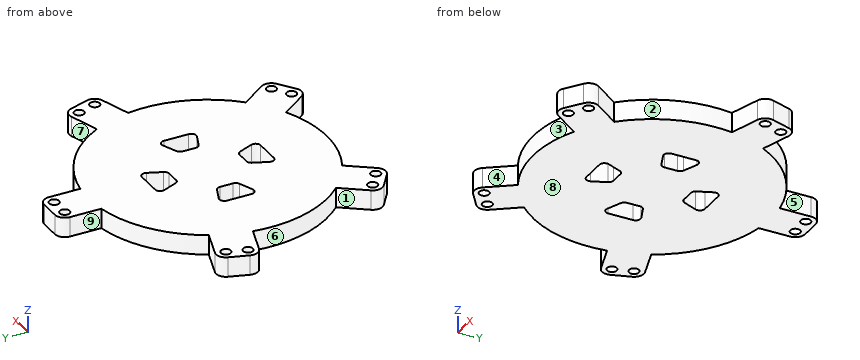
from build123d import *

# Parameters (mm, degrees)
F0_R     = 1.5875
F1_DEPTH = 6.3754
F3_DEPTH = 6.3764


with BuildPart() as f1:
    # F0 (on Top) → F1 (new body)
    with BuildSketch(Plane.XY):
        with BuildLine():
            Line((-6.35, 47.625), (-6.35, 37.567107))
            ThreePointArc((-6.35, 37.567107), (-22.394618, 30.823547), (-33.766184, 17.648083))
            Line((-33.766184, 17.648083), (-43.331809, 20.756143))
            ThreePointArc((-43.331809, 20.756143), (-45.754357, 20.565485), (-47.332542, 18.717668))
            Line((-47.332542, 18.717668), (-49.2948, 12.678459))
            ThreePointArc((-49.2948, 12.678459), (-49.104141, 10.25591), (-47.256325, 8.677725))
            Line((-47.256325, 8.677725), (-37.690699, 5.569665))
            ThreePointArc((-37.690699, 5.569665), (-36.235253, -11.773547), (-27.218649, -26.659991))
            Line((-27.218649, -26.659991), (-33.130531, -34.796998))
            ThreePointArc((-33.130531, -34.796998), (-33.697812, -37.159896), (-32.42812, -39.231845))
            Line((-32.42812, -39.231845), (-27.290862, -42.964281))
            ThreePointArc((-27.290862, -42.964281), (-24.927964, -43.531563), (-22.856015, -42.261871))
            Line((-22.856015, -42.261871), (-16.944133, -34.124864))
            ThreePointArc((-16.944133, -34.124864), (0, -38.1), (16.944133, -34.124864))
            Line((16.944133, -34.124864), (22.856015, -42.261871))
            ThreePointArc((22.856015, -42.261871), (24.927964, -43.531563), (27.290862, -42.964281))
            Line((27.290862, -42.964281), (32.42812, -39.231845))
            ThreePointArc((32.42812, -39.231845), (33.697812, -37.159896), (33.130531, -34.796998))
            Line((33.130531, -34.796998), (27.218649, -26.659991))
            ThreePointArc((27.218649, -26.659991), (36.235253, -11.773547), (37.690699, 5.569665))
            Line((37.690699, 5.569665), (47.256325, 8.677725))
            ThreePointArc((47.256325, 8.677725), (49.104141, 10.25591), (49.2948, 12.678459))
            Line((49.2948, 12.678459), (47.332542, 18.717668))
            ThreePointArc((47.332542, 18.717668), (45.754357, 20.565485), (43.331809, 20.756143))
            Line((43.331809, 20.756143), (33.766184, 17.648083))
            ThreePointArc((33.766184, 17.648083), (22.394618, 30.823547), (6.35, 37.567107))
            Line((6.35, 37.567107), (6.35, 47.625))
            ThreePointArc((6.35, 47.625), (5.420064, 49.870064), (3.175, 50.8))
            Line((3.175, 50.8), (-3.175, 50.8))
            ThreePointArc((-3.175, 50.8), (-5.420064, 49.870064), (-6.35, 47.625))
        make_face()
        with Locations((-25.424644, -40.395653)):
            Circle(F0_R, mode=Mode.SUBTRACT)
        with Locations((-30.561902, -36.663216)):
            Circle(F0_R, mode=Mode.SUBTRACT)
        with Locations((25.424644, -40.395653)):
            Circle(F0_R, mode=Mode.SUBTRACT)
        with Locations((30.561902, -36.663216)):
            Circle(F0_R, mode=Mode.SUBTRACT)
        with Locations((-46.275196, 11.69733)):
            Circle(F0_R, mode=Mode.SUBTRACT)
        with Locations((-44.312938, 17.736539)):
            Circle(F0_R, mode=Mode.SUBTRACT)
        with Locations((-3.175, 47.625)):
            Circle(F0_R, mode=Mode.SUBTRACT)
        with Locations((46.275196, 11.69733)):
            Circle(F0_R, mode=Mode.SUBTRACT)
        with Locations((44.312938, 17.736539)):
            Circle(F0_R, mode=Mode.SUBTRACT)
        with Locations((3.175, 47.625)):
            Circle(F0_R, mode=Mode.SUBTRACT)
    extrude(amount=F1_DEPTH)

    # F2 (on face) → F3 (cut, through all)
    with BuildSketch(Plane.XY.offset(6.3754)):
        with BuildLine():
            Line((3.984938, 19.05), (0, 19.05))
            Line((0, 19.05), (-3.984938, 19.05))
            ThreePointArc((-3.984938, 19.05), (-5.303035, 18.347246), (-5.454143, 16.861174))
            Line((-5.454143, 16.861174), (-3.578628, 12.278771))
            ThreePointArc((-3.578628, 12.278771), (-2.994169, 11.562), (-2.109423, 11.292597))
            Line((-2.109423, 11.292597), (0, 11.292597))
            Line((0, 11.292597), (2.109423, 11.292597))
            ThreePointArc((2.109423, 11.292597), (2.994169, 11.562), (3.578628, 12.278771))
            Line((3.578628, 12.278771), (5.454143, 16.861174))
            ThreePointArc((5.454143, 16.861174), (5.303035, 18.347246), (3.984938, 19.05))
        make_face()
        with BuildLine():
            Line((19.05, -3.984938), (19.05, 0))
            Line((19.05, 0), (19.05, 3.984938))
            ThreePointArc((19.05, 3.984938), (18.347246, 5.303035), (16.861174, 5.454143))
            Line((16.861174, 5.454143), (12.278771, 3.578628))
            ThreePointArc((12.278771, 3.578628), (11.562, 2.994169), (11.292597, 2.109423))
            Line((11.292597, 2.109423), (11.292597, 0))
            Line((11.292597, 0), (11.292597, -2.109423))
            ThreePointArc((11.292597, -2.109423), (11.562, -2.994169), (12.278771, -3.578628))
            Line((12.278771, -3.578628), (16.861174, -5.454143))
            ThreePointArc((16.861174, -5.454143), (18.347246, -5.303035), (19.05, -3.984938))
        make_face()
        with BuildLine():
            Line((-3.984938, -19.05), (0, -19.05))
            Line((0, -19.05), (3.984938, -19.05))
            ThreePointArc((3.984938, -19.05), (5.303035, -18.347246), (5.454143, -16.861174))
            Line((5.454143, -16.861174), (3.578628, -12.278771))
            ThreePointArc((3.578628, -12.278771), (2.994169, -11.562), (2.109423, -11.292597))
            Line((2.109423, -11.292597), (0, -11.292597))
            Line((0, -11.292597), (-2.109423, -11.292597))
            ThreePointArc((-2.109423, -11.292597), (-2.994169, -11.562), (-3.578628, -12.278771))
            Line((-3.578628, -12.278771), (-5.454143, -16.861174))
            ThreePointArc((-5.454143, -16.861174), (-5.303035, -18.347246), (-3.984938, -19.05))
        make_face()
        with BuildLine():
            Line((-19.05, 3.984938), (-19.05, 0))
            Line((-19.05, 0), (-19.05, -3.984938))
            ThreePointArc((-19.05, -3.984938), (-18.347246, -5.303035), (-16.861174, -5.454143))
            Line((-16.861174, -5.454143), (-12.278771, -3.578628))
            ThreePointArc((-12.278771, -3.578628), (-11.562, -2.994169), (-11.292597, -2.109423))
            Line((-11.292597, -2.109423), (-11.292597, 0))
            Line((-11.292597, 0), (-11.292597, 2.109423))
            ThreePointArc((-11.292597, 2.109423), (-11.562, 2.994169), (-12.278771, 3.578628))
            Line((-12.278771, 3.578628), (-16.861174, 5.454143))
            ThreePointArc((-16.861174, 5.454143), (-18.347246, 5.303035), (-19.05, 3.984938))
        make_face()
    extrude(amount=-F3_DEPTH, mode=Mode.SUBTRACT)


solid = f1.part
The listing builds one solid part. Answer for the finished solid, in the listing's coordinates (mm). Face numbers are marked on the shaded views. A direction names the side the tool comes from. Give positions to 0.01 mm unless a question says otherwise; leave off trailing zeros. Order: outer loops, then holes, each group sorted by start corner. A loop starts at its lowest first (then second) coordinate and runs counter-clockwise, first axis right, second up. Notation, with made-up numbers: (78, 22) -> (127, 22) arc R17 ccw to (127, 36) -> close; hole circle Ø1 at (63.25, -32.75). An arc over 180 degrees is marked (long way). Put each result on its own line as item: value.
Item 1: For the marked faces 5, 6, 7, 8 and 9, determine the directions among +Z, -Z, +X, -X, +Y, -Y from which every point of the face is accessible in a straight line to the end or side of a thin tool.
Established:
face 5: +Z, -Z, +X, +Y
face 6: +Z, -Z, -X
face 7: +Z, -Z, +Y
face 8: -Z, +X, -X, +Y, -Y
face 9: +Z, -Z, -X, +Y
Item 2: A cutting plane is placed at D-D on y = -22. Give the vertices of the cut face in (x, z).
Established:
outline: (-31.11, 0) -> (31.11, 0) -> (31.11, 6.38) -> (-31.11, 6.38) -> close
Item 3: A cutting plane is placed at C-C on z = 3.5. Count the separate pieces of the cut face and the enclosed holes in it, plus the area to 3 significant figures.
Established:
separate pieces: 1
enclosed holes: 14
area: 4,990 mm^2
Item 4: A cutting plane is placed at B-B on y = 42.5. Give the vertices of the cut face in (x, z), plus the area to 3 significant figures.
Established:
outline: (-6.35, 0) -> (6.35, 0) -> (6.35, 6.38) -> (-6.35, 6.38) -> close
area: 81.0 mm^2
Item 5: A cutting plane is placed at A-A on x = 15. Give the vertices of the cut face in (y, z), plus the area to 3 significant figures.
Established:
outline: (-35.02, 0) -> (-4.69, 0) -> (-4.69, 6.38) -> (-35.02, 6.38) -> close; (4.69, 0) -> (35.02, 0) -> (35.02, 6.38) -> (4.69, 6.38) -> close
area: 387 mm^2
Item 6: Given P1, Ø1, axis at x = 1.5, z = 2.5, coming from the -Y side; P2, Ø2, axis at y = 0, z = 2.5, coming from the -X side; P3, Ø3.5, axis at y = -1, z = 2.5, coming from the +X side, each flat-ended and moving along its own axis, determine where each tip first touches the part or whether it passes through.
Established:
P1: stops at y = -38.09
P2: stops at x = -38.1
P3: stops at x = 38.1
Item 7: For a pull along X with two mould halves and no side action, classify the marked faces 1, 2, 3 and 4 as released by +X, released by -X, zero draft, split by the parting line, or undercut.
Established:
face 1: released by -X
face 2: released by +X
face 3: undercut
face 4: undercut
Item 8: Straight lines are drawn through the part: line 1 (X direction, y = 1, z = 5.5); line 2 (Y direction, x = -2, z = 3.75); line 3 (Y direction, x = -45, z = 0.5). For each, find the intervals that lie inside material, in ascending order.
Established:
line 1: x = -38.09 to -19.05, -11.29 to 11.29, 19.05 to 38.09
line 2: y = -38.05 to -19.05, -11.29 to 11.29, 19.05 to 46.56, 48.69 to 50.8
line 3: y = 7.94 to 10.75, 12.64 to 16.31, 19.17 to 20.84
